from build123d import *

# Parameters (mm, degrees)
F0_W     = 55.0028979778
F0_H     = 25.8127627894
F0_R     = 2.8370403088
F1_DEPTH = 3
F2_R     = 5


with BuildPart() as f1:
    # F0 (on Top) → F1 (new body)
    with BuildSketch(Plane.XY):
        with Locations((-11.7194391787, -5.7870582677)):
            Rectangle(F0_W, F0_H)
        with BuildLine():
            Line((-16.200212838, 2.2999899667), (-16.200212838, -15.1974810287))
            Line((-16.200212838, -15.1974810287), (-20.9144581423, -15.1974810287))
            Line((-20.9144581423, -15.1974810287), (-28.5277153843, -1.9623617991))
            Line((-28.5277153843, -1.9623617991), (-28.6349443596, -1.9623617991))
            add(Edge.make_bspline(
                [(-28.6349443596, -1.9623617991), (-28.405167984, -5.4664515257), (-28.405167984, -6.9638275728)],
                knots=[0, 0, 0, 1, 1, 1], degree=2))
            Line((-28.405167984, -6.9638275728), (-28.405167984, -15.1974810287))
            Line((-28.405167984, -15.1974810287), (-31.721607004, -15.1974810287))
            Line((-31.721607004, -15.1974810287), (-31.721607004, 2.2999899667))
            Line((-31.721607004, 2.2999899667), (-27.041828156, 2.2999899667))
            Line((-27.041828156, 2.2999899667), (-19.443889339, -10.8049226501))
            Line((-19.443889339, -10.8049226501), (-19.3596380013, -10.8049226501))
            add(Edge.make_bspline(
                [(-19.3596380013, -10.8049226501), (-19.5396294954, -7.3927434738), (-19.5396294954, -5.9834483706)],
                knots=[0, 0, 0, 1, 1, 1], degree=2))
            Line((-19.5396294954, -5.9834483706), (-19.5396294954, 2.2999899667))
            Line((-19.5396294954, 2.2999899667), (-16.200212838, 2.2999899667))
        make_face(mode=Mode.SUBTRACT)
        Polygon((-7.403607262, -15.1974810287), (-11.2829984019, -15.1974810287), (-4.7113940622, -0.8364575591), (-13.3394969628, -0.8364575591), (-13.3394969628, 2.2770123292), (-0.7860476472, 2.2770123292), (-0.7860476472, -0.0475586698), align=None, mode=Mode.SUBTRACT)
        Polygon((6.1111208051, -15.3139589772), (-4.0005319752, -15.1974810287), (2.923307009, 0), (2.923307009, 2.1986574866), (6.1111208051, 2.1986574866), align=None, mode=Mode.SUBTRACT)
        with Locations((11.1188692972, 2.7992387768)):
            Circle(F0_R, mode=Mode.SUBTRACT)
    extrude(amount=F1_DEPTH)

    # F2
    f2_edges = [f1.edges().sort_by_distance(p)[0] for p in [
        (-39.220888, 7.119323, 1.5),
        (-39.220888, -18.69344, 1.5),
        (15.78201, 7.119323, 1.5),
        (15.78201, -18.69344, 1.5),
    ]]
    fillet(f2_edges, radius=F2_R)


solid = f1.part
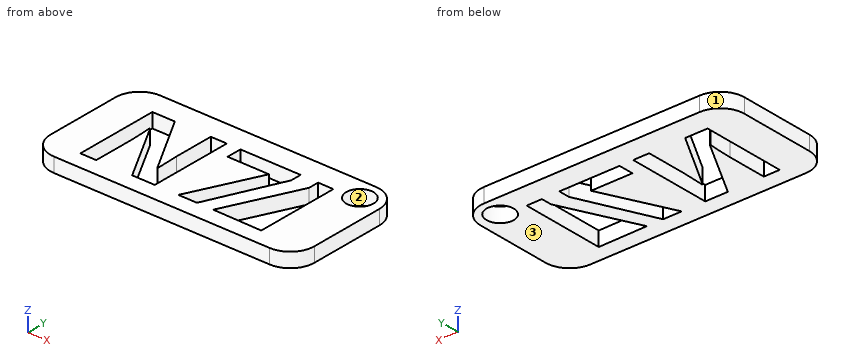
Can you work these out from the model? Positions are in its coordinate system, mm. Face numbers are marked on the shaded views. Round coordinates to 2 decimals unless told otherwise and drop trailing zeros. Loops run counter-clockwise (first coordinate to the right, second up) from the corner with the lowest first, then second, coordinate; pieces in that order, holes last. Notation, with made-up numbers: (-15.5, 52.25) - (22.5, 52.25) arc R25 cw to (22.5, 75.25) - close; hole circle Ø2 at (20, 53.25). An arc over 180 degrees is marked (long way). Answer in a Markdown table with one row per item. Add a question column.
Q1. I want a section at A-A on x = -12. List the corners of the cut face in (y, z) for me.
Q2. We'd pull the mould along Y, two halves only. Please class the marked faces 1, 2 and 3: pulls with the +Y half, pulls with the -Y half, needs draft (parallel to the pull), parting line crosses it, or undercut.
Q3. I need wall thicknesses on L1, parallel to Y at x = -1, z = 0.3; L2, parallel to Y at x = -12, z = 0.15; L3, parallel to X at y = -6, z = 1.2. Which ranges of each line are inside material? Lowest first, please.
Q4. For pin 1 Ø4 at (x, y) = (-2, -6.5) entering from -Z; pin 2 Ø1.5 at (y, z) = (-16, 0.5) entering from +X, each with a flat end and sliding along its axis, tell me the tip position at first contact or that it passes through.
Q5. I want a section at B-B on x = -25.5. List the corners of the cut face in (y, z) for me, and give its area (3 significant figures).
Q6. I want a section at C-C on y = -9.25. Count the separate pieces of the cut face and the enclosed holes in it, and give its area (3 significant figures).
A:
| question | item | result |
|---|---|---|
| 1 | outline | (-18.69, 0) - (-0.84, 0) - (-0.84, 3) - (-18.69, 3) - close; (2.28, 0) - (7.12, 0) - (7.12, 3) - (2.28, 3) - close |
| 2 | face 1 | pulls with the +Y half |
| 2 | face 2 | undercut |
| 2 | face 3 | needs draft |
| 3 | L1 | -18.69 to -15.23, -8.61 to -0.54, 2.28 to 7.12 |
| 3 | L2 | -18.69 to -0.84, 2.28 to 7.12 |
| 3 | L3 | -39.22 to -31.72, -28.42 to -26.21, -22.23 to -19.54, -16.2 to -7.07, -3.39 to 0.19, 6.11 to 15.78 |
| 4 | pin 1 | z = 0 |
| 4 | pin 2 | x = 15.53 |
| 5 | outline | (-18.69, 0) - (-7.23, 0) - (-7.23, 3) - (-18.69, 3) - close; (-0.36, 0) - (7.12, 0) - (7.12, 3) - (-0.36, 3) - close |
| 5 | area | 56.8 mm^2 |
| 6 | separate pieces | 6 |
| 6 | enclosed holes | 0 |
| 6 | area | 99.9 mm^2 |
